Design review of the part built by this model. Coordinates are the model's own, in mm. Face numbers are marked on the shaded views. A direction names the side the tool comes from. Give positions to 0.01 mm unless a question says otherwise; leave off trailing zeros. Write each loop counter-clockwise with the first axis right and the second up, starting at its lowest first coordinate (ties: lowest second). Pieces come first, ordered by that corner, then holes. Notation, with made-up numbers: (58, 63.5) -> (74, 63.5) arc R35 ccw to (74, 95.5) -> close; hole circle Ø7 at (72, 79.5). An arc over 180 degrees is marked (long way). Answer as a JSON object with one key per item and string values.
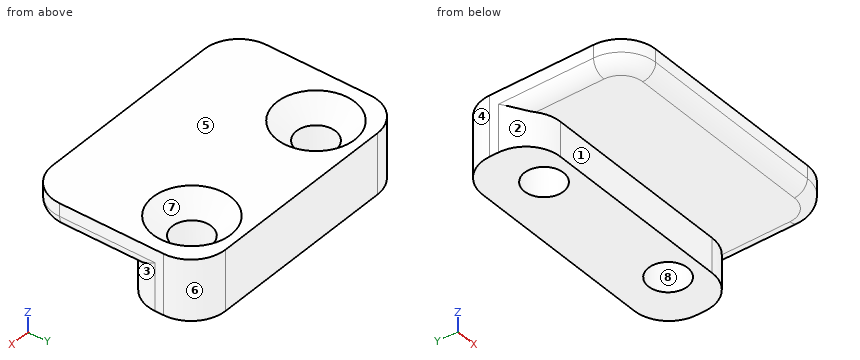
```python
from build123d import *

# Parameters (mm, degrees)
F1_DEPTH       = 15
F3_D           = 4.5
F3_CSINK_D     = 9
F3_CSINK_ANGLE = 90
F4_R           = 4
F5_R           = 1.5


with BuildPart() as f1:
    # F0 (on Right) → F1 (new body, symmetric)
    with BuildSketch(Plane.YZ):
        Polygon((0, 4), (0, 0), (9, 0), (9, 7), (-11, 7), (-11, 4), align=None)
    extrude(amount=F1_DEPTH, both=True)

    # F3 (through all)
    with Locations(Plane.XY.offset(7)):
        with Locations((-9, 3.5), (9, 3.5)):
            CounterSinkHole(F3_D / 2, F3_CSINK_D / 2, counter_sink_angle=F3_CSINK_ANGLE)

    # F4
    f4_edges = [f1.edges().sort_by_distance(p)[0] for p in [
        (15, -11, 5.5),
        (-15, -11, 5.5),
        (15, 0, 2),
        (-15, 0, 2),
        (-15, 9, 3.5),
        (15, 9, 3.5),
    ]]
    fillet(f4_edges, radius=F4_R)

    # F5
    f5_edges = [f1.edges().sort_by_distance(p)[0] for p in [
        (-15, -3.5, 4),
    ]]
    fillet(f5_edges, radius=F5_R)


solid = f1.part
```
(1) We need section A-A, the plane x = -9. State the section outline as (y, z) points.
Here are the results:
{"outline": "(-11, 5.5) arc R1.5 ccw to (-9.5, 4) -> (0, 4) -> (0, 0) -> (1.25, 0) -> (1.25, 4.75) -> (-1, 7) -> (-11, 7) -> close; (5.75, 0) -> (9, 0) -> (9, 7) -> (8, 7) -> (5.75, 4.75) -> close"}
(2) We need section B-B, the plane z = 3. State the section outline as (x, y) points.
Here are the results:
{"outline": "(-15, 4) arc R4 ccw to (-11, 0) -> (11, 0) arc R4 ccw to (15, 4) -> (15, 5) arc R4 ccw to (11, 9) -> (-11, 9) arc R4 ccw to (-15, 5) -> close; hole circle Ø4.5 at (-9, 3.5); hole circle Ø4.5 at (9, 3.5)"}
(3) The part is to be moulded in two halves that separate along X. For the marked faces 5, 6, 7 and 8, say which applies: +X half, -X half, draft (parallel to the pull), parting line (faces both ways), or undercut.
Here are the results:
{"face 5": "draft", "face 6": "+X half", "face 7": "undercut", "face 8": "undercut"}
(4) For the marked faces 1, 2, 3 and 4, list the 3-axis set-ups (+Z, -Z, +X, -X, +Y, -Y) from which the entire face can be reached by the end or side of a thin tool; tool diameter is ignored.
Here are the results:
{"face 1": "-Z, +X, -X, -Y", "face 2": "-Z, -X, -Y", "face 3": "-Z, +X, -Y", "face 4": "+Z, -Z, -X, +Y"}
(5) We need section D-D, the plane x = -1.5. State the section outline as (y, z) points, then the cut area to 3 significant figures.
Here are the results:
{"outline": "(-11, 5.5) arc R1.5 ccw to (-9.5, 4) -> (0, 4) -> (0, 0) -> (9, 0) -> (9, 7) -> (-11, 7) -> close", "area": "95.5 mm²"}
(6) For line 1 along Y through (x, z) = (-9, 3.75); line 2 along X through (y, z) = (3.5, 2.5); line 3 along X through (y, z) = (2.25, 2.75), list the stretches that pass through material, from the lowest coordinate up.
Here are the results:
{"line 1": "y = 0 to 1.25, 5.75 to 9", "line 2": "x = -14.97 to -11.25, -6.75 to 6.75, 11.25 to 14.97", "line 3": "x = -14.6 to -10.87, -7.13 to 7.13, 10.87 to 14.6"}
(7) Clearance check with a flat-ended pin moving along its axis: pin 1 (8.5 mm diameter, centred on x = 4.5, y = -7, fed in from -Z). State where the tip first meets the part, or that it passes through.
Here are the results:
{"pin 1": "stops at z = 4"}
(8) We need section C-C, the plane y = 3.5. State the section outline as (x, z) points, then the cut area to 3 significant figures.
Here are the results:
{"outline": "(-15, 5.5) arc R1.5 ccw to (-14.97, 5.19) -> (-14.97, 0) -> (-11.25, 0) -> (-11.25, 4.75) -> (-13.5, 7) -> (-15, 7) -> close; (-6.75, 0) -> (6.75, 0) -> (6.75, 4.75) -> (4.5, 7) -> (-4.5, 7) -> (-6.75, 4.75) -> close; (11.25, 0) -> (14.97, 0) -> (14.97, 5.19) arc R1.5 ccw to (15, 5.5) -> (15, 7) -> (13.5, 7) -> (11.25, 4.75) -> close", "area": "137 mm²"}
